```python
from build123d import *

# Parameters (mm, degrees)
SKETCH1_R           = 1.6
BOSS_EXTRUDE1_DEPTH = 4.7625


with BuildPart() as part:
    # Sketch1 → Boss-Extrude1 (new body)
    with BuildSketch(Plane(origin=(0, 0, 0), x_dir=(1, 0, 0), z_dir=(0, 1, 0))):
        Polygon((0, 0), (61.9, 0), (66.6625, 0), (66.6625, 5.6), (61.9, 5.6), (61.9, 11.2), (66.6625, 11.2), (66.6625, 16.8), (61.9, 16.8), (61.9, 22.4), (66.6625, 22.4), (66.6625, 28), (61.9, 28), (61.9, 33.6), (66.6625, 33.6), (66.6625, 39.2), (61.9, 39.2), (61.9, 44.8), (66.6625, 44.8), (66.6625, 50.4), (61.9, 50.4), (61.9, 56), (66.6625, 56), (66.6625, 61.6), (61.9, 61.6), (61.9, 67.2), (66.6625, 67.2), (66.6625, 72.8), (61.9, 72.8), (61.9, 78.4), (66.6625, 78.4), (66.6625, 84), (61.9, 84), (0, 84), align=None)
        with Locations((2.16, 81.16)):
            Circle(SKETCH1_R, mode=Mode.SUBTRACT)
        with Locations((2.16, 2.84)):
            Circle(SKETCH1_R, mode=Mode.SUBTRACT)
        with Locations((59.74, 2.84)):
            Circle(SKETCH1_R, mode=Mode.SUBTRACT)
        with Locations((59.74, 81.16)):
            Circle(SKETCH1_R, mode=Mode.SUBTRACT)
    extrude(amount=BOSS_EXTRUDE1_DEPTH)


solid = part.part
```
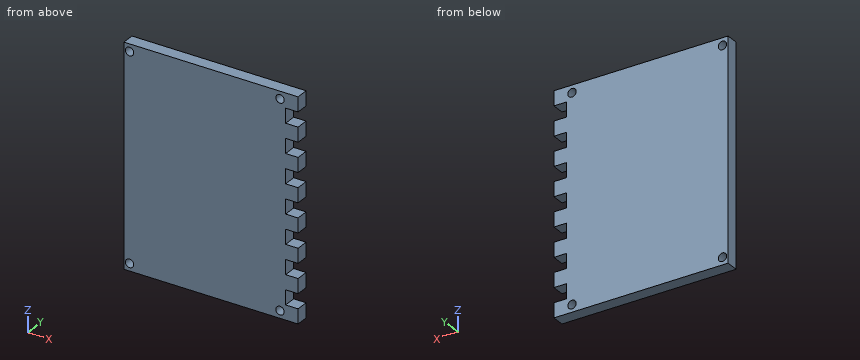
Check sheet for the modelled part. Datum: model origin and axes. Units: mm. Round coordinates to 2 decimals unless told otherwise and drop trailing zeros. Order: outer loops, then holes, each group sorted by start corner. A loop starts at its lowest first (then second) coordinate and runs counter-clockwise, first axis right, second up. Notation, with made-up numbers: (8, 38.25) - (63, 38.25) arc R17 cw to (63, 48.25) - close; hole circle Ø6 at (0.25, 83). An arc over 180 degrees is marked (long way). Answer as CSV lines item,"result". Start each with the question number.
1) Depth check by flat-ended pin: pin 1 (1.4 mm diameter, centred on y = 3, z = -30.5, fed in from +X). Enter the tip coordinate at first touch or a pass-through.
2) Section check C-C (y = 3.45). Give the number of separate pieces and of enclosed holes in the cut face, then the cut area to 3 significant figures.
3) Section check D-D (z = -29). Record the cut outline in (x, y), then the cut area to 3 significant figures.
4) Section check B-B (z = -81.16). Record the cut outline in (x, y), then the cut area to 3 significant figures.
5) Section check A-A (x = 59.74). Record the cut outline in (y, z).
6) Scan lines: probe 1 along Z at (x, y) = (59.74, 3.4); probe 2 along X at (y, z) = (2.55, -2.84); probe 3 along X at (y, z) = (2.5, -54). Record each from-to range of solid material in increasing order.
Determined:
1,pin 1,"x = 61.9"
2,separate pieces,"1"
2,enclosed holes,"4"
2,area,"5,380 mm^2"
3,outline,"(0, 0) - (61.9, 0) - (61.9, 4.76) - (0, 4.76) - close"
3,area,"295 mm^2"
4,outline,"(0, 0) - (0.56, 0) - (0.56, 4.76) - (0, 4.76) - close; (3.76, 0) - (58.14, 0) - (58.14, 4.76) - (3.76, 4.76) - close; (61.34, 0) - (66.66, 0) - (66.66, 4.76) - (61.34, 4.76) - close"
4,area,"287 mm^2"
5,outline,"(0, -84) - (4.76, -84) - (4.76, -82.76) - (0, -82.76) - close; (0, -79.56) - (4.76, -79.56) - (4.76, -4.44) - (0, -4.44) - close; (0, -1.24) - (4.76, -1.24) - (4.76, 0) - (0, 0) - close"
6,probe 1,"-84 to -82.76, -79.56 to -4.44, -1.24 to 0"
6,probe 2,"0 to 0.56, 3.76 to 58.14, 61.34 to 66.66"
6,probe 3,"0 to 61.9"
